Read the model definition and answer for the solid it produces. Units are mm, in the model's axes. A direction names the side the tool comes from. Coordinates: 2 decimals unless noted, no trailing zeros. Write each loop counter-clockwise with the first axis right and the second up, starting at its lowest first coordinate (ties: lowest second). Pieces come first, ordered by that corner, then holes. Notation, with made-up numbers: (-32, 31) -> (-9, 31) arc R29 cw to (-9, 69) -> close; hole circle Ø6 at (88, 60.25). An arc over 180 degrees is marked (long way). Return JSON: item names as keys, results as strings.
from build123d import *

# Parameters (mm, degrees)
F2_ANGLE_BACK = 77.5
F2_ANGLE      = 155
F3_SIZE       = 1
F4_R          = 1


with BuildPart() as f2:
    # F1 (on Right) → F2 (revolve)
    with BuildSketch(Plane.YZ, mode=Mode.PRIVATE) as f2_sk:
        Polygon((754.5, -22), (754.5, 0), (751.5, 0), (751.5, -25), (792.5, -25), (792.5, 0), (789.5, 0), (789.5, -22), align=None)
    revolve(f2_sk.sketch.rotate(Axis((0, 0, -26.4390427619), (0, 0, -1)), -F2_ANGLE_BACK), axis=Axis((0, 0, -26.4390427619), (0, 0, -1)), revolution_arc=F2_ANGLE)

    # F3
    f3_edges = [f2.edges().sort_by_distance(p)[0] for p in [
        (0, 789.5, 0),
        (0, 792.5, 0),
        (0, 751.5, 0),
        (0, 754.5, 0),
    ]]
    chamfer(f3_edges, length=F3_SIZE)

    # F4
    f4_edges = [f2.edges().sort_by_distance(p)[0] for p in [
        (0, 789.5, -22),
        (0, 754.5, -22),
    ]]
    fillet(f4_edges, radius=F4_R)


solid = f2.part
1. Consider L1, parallel to X at y = 270, z = -18.5; L2, parallel to X at y = 495, z = -21; L3, parallel to X at y = 310, z = -23.5. Determine where each line is inside the solid, lowest interval first.
Taken from the geometry:
{"L1": "x = -745.09 to -741.9, -704.54 to -701.32, 701.32 to 704.54, 741.9 to 745.09", "L2": "x = -618.9 to -615.05, -569.43 to -565.44, 565.44 to 569.43, 615.05 to 618.9", "L3": "x = -729.35 to -684.58, 684.58 to 729.35"}
2. For a pull along Y with two mould halves and no side action, classify faces 3 (the face through (20, 760, -22)), 4 (the face through (-14.95, 789.36, -11.14)), 5 (the face through (13, 766, -25)), 6 (the face through (-15.007, 792.358, -12.832)) as +Y half, -Y half, draft (parallel to the pull), parting line (faces both ways), or undercut.
Taken from the geometry:
{"face 3": "undercut", "face 4": "undercut", "face 5": "draft", "face 6": "+Y half"}
3. The part is cut by section A-A (z = -7.5). Determine the outline of the cut face in (x, y).
Taken from the geometry:
{"outline": "(-773.71, 171.53) -> (-770.79, 170.88) arc R789.5 cw to (770.79, 170.88) -> (773.71, 171.53) arc R792.5 ccw to start; (-736.62, 163.3) -> (-733.69, 162.65) arc R751.5 cw to (733.69, 162.65) -> (736.62, 163.3) arc R754.5 ccw to start"}
4. Flat-ended cylindrical pins translate along their axes: pin 1 Ø1 at (x, z) = (-550.5, -15.5) entering from -Y; pin 2 Ø2 at (x, z) = (146.5, -3) entering from -Y; pin 3 Ø3 at (x, z) = (-488, -4) entering from -Y. Find the tip coordinate at first contact, or state that the pin passes through.
Taken from the geometry:
{"pin 1": "stops at y = 511.03", "pin 2": "stops at y = 736.88", "pin 3": "stops at y = 570.21"}
5. A tool of negligible diameter and unlimited length cuts with its end or side. For faces 1 (the face through (-14.233, 751.525, -0.84)), 2 (the face through (-14.287, 754.365, -10.86)), from which of +Z, -Z, +X, -X, +Y, -Y can it reach the whole face along a straight path? Write none if from no direction.
Taken from the geometry:
{"face 1": "+Z, -Y", "face 2": "+Z"}
